The listing builds one solid part. Answer for the finished solid, in the listing's coordinates (mm). A direction names the side the tool comes from. Round coordinates to 2 decimals unless told otherwise and drop trailing zeros. Order: outer loops, then holes, each group sorted by start corner. A loop starts at its lowest first (then second) coordinate and runs counter-clockwise, first axis right, second up. Notation, with made-up numbers: (68, 27.25) -> (118, 27.25) arc R10 ccw to (118, 35.25) -> close; hole circle Ø11 at (38, 8). An arc over 180 degrees is marked (long way). Answer in a Markdown table with one row per item. Add a question column.
```python
from build123d import *

# Parameters (mm, degrees)
SKETCH1_R           = 10
BOSS_EXTRUDE1_DEPTH = 30
SKETCH2_W           = 6
SKETCH2_H           = 3.26
BOSS_EXTRUDE2_DEPTH = 9


with BuildPart() as part:
    # Sketch1 → Boss-Extrude1 (new body, symmetric)
    with BuildSketch(Plane.XY):
        Circle(SKETCH1_R)
    extrude(amount=BOSS_EXTRUDE1_DEPTH, both=True)

    # Sketch2 → Boss-Extrude2 (add)
    with BuildSketch(Plane.XY.offset(30)):
        with Locations((0, 11.115019423)):
            Rectangle(SKETCH2_W, SKETCH2_H)
    boss_extrude2 = extrude(amount=-BOSS_EXTRUDE2_DEPTH)

    # Mirror1: Boss-Extrude2 across plane
    add(boss_extrude2.mirror(Plane.XY))


solid = part.part
```
1. The part is cut by section D-D (y = -6.75). Give the vertices of the cut face in (x, z).
2. Straight lines are drawn through the part: line 1 along Y through (x, z) = (0, -13.5); line 2 along X through (y, z) = (9.75, 27.5); line 3 along X through (y, z) = (-0.5, -1). For each, find the intervals that lie inside material, in ascending order.
3. The part is cut by section B-B (x = 0). Give the vertices of the cut face in (y, z).
4. Each of these flat-tipped pins is pushed along its axis until it touches: pin 1 (2 mm diameter, centred on y = -5, z = 14.5, fed in from +X); pin 2 (1 mm diameter, centred on y = 11, z = 24, fed in from -X); pin 3 (3 mm diameter, centred on x = 3.5, z = 16.5, fed in from +Y). Where does it stop, or does it pass through?
5. For faces 5 (the flat face through (-3, 11, -26)), 6 (the flat face through (0, 12.745, 26)), 7 (the flat face through (3, 11, 26)), determine the directions among +Z, -Z, +X, -X, +Y, -Y from which every point of the face is accessible in a straight line to the end or side of a thin tool.
6. The mould has two halves that part along Z. Classify faces 1 (the flat face through (0, 2, -30)), 2 (the flat face through (0, 2, 30)), 3 (the flat face through (-3, 11, 26)), 4 (the flat face through (0, 11, 21)): released by +Z, released by -Z, zero draft, split by the parting line, or undercut.
7. The part is cut by section C-C (z = -14.5). Give the vertices of the cut face in (x, y), then the cut area to 3 significant figures.
8. The part is cut by section A-A (y = 10.75). Give the vertices of the cut face in (x, z), then the cut area to 3 significant figures.
Report:
| question | item | result |
|---|---|---|
| 1 | outline | (-7.38, -30) -> (7.38, -30) -> (7.38, 30) -> (-7.38, 30) -> close |
| 2 | line 1 | y = -10 to 10 |
| 2 | line 2 | x = -3 to 3 |
| 2 | line 3 | x = -9.99 to 9.99 |
| 3 | outline | (-10, -30) -> (12.75, -30) -> (12.75, -21) -> (10, -21) -> (10, 21) -> (12.75, 21) -> (12.75, 30) -> (-10, 30) -> close |
| 4 | pin 1 | stops at x = 9.17 |
| 4 | pin 2 | stops at x = -3 |
| 4 | pin 3 | stops at y = 9.8 |
| 5 | face 5 | +Z, -Z, -X, +Y |
| 5 | face 6 | +Z, -Z, +X, -X, +Y |
| 5 | face 7 | +Z, -Z, +X, +Y |
| 6 | face 1 | released by -Z |
| 6 | face 2 | released by +Z |
| 6 | face 3 | zero draft |
| 6 | face 4 | undercut |
| 7 | outline | circle Ø20 at (0, 0) |
| 7 | area | 314 mm^2 |
| 8 | outline | (-3, -30) -> (3, -30) -> (3, -21) -> (-3, -21) -> close; (-3, 21) -> (3, 21) -> (3, 30) -> (-3, 30) -> close |
| 8 | area | 108 mm^2 |
